```python
from build123d import *

# Parameters (mm, degrees)
SKETCH1_R                = 15
SKETCH1_R_2              = 7.5
BOSS_EXTRUDE1_DEPTH      = 160
BOSS_EXTRUDE1_DEPTH_BACK = 160
SKETCH2_R                = 3.1
CUT_EXTRUDE1_DEPTH       = 16


with BuildPart() as part:
    # Sketch1 → Boss-Extrude1 (new body, two sides)
    with BuildSketch(Plane.XY) as boss_extrude1_sk:
        Circle(SKETCH1_R)
        Circle(SKETCH1_R_2, mode=Mode.SUBTRACT)
    extrude(amount=BOSS_EXTRUDE1_DEPTH)
    extrude(boss_extrude1_sk.sketch, amount=-BOSS_EXTRUDE1_DEPTH_BACK)

    # Sketch2 → Cut-Extrude1 (cut, through all)
    with BuildSketch(Plane(origin=(0, 0, 0), x_dir=(1, 0, 0), z_dir=(0, 1, 0))):
        with Locations((0, -145)):
            Circle(SKETCH2_R)
    cut_extrude1 = extrude(amount=CUT_EXTRUDE1_DEPTH, mode=Mode.SUBTRACT)

    # Mirror1: Cut-Extrude1 across plane
    add(cut_extrude1.mirror(Plane.XY), mode=Mode.SUBTRACT)


solid = part.part
```
The model under review builds one solid part; all positions refer to its coordinate system, in mm. Round coordinates to 2 decimals unless told otherwise and drop trailing zeros. Loops run counter-clockwise (first coordinate to the right, second up) from the corner with the lowest first, then second, coordinate; pieces in that order, holes last. Notation, with made-up numbers: (75, -24.5) -> (123, -24.5) arc R12 ccw to (123, -13.5) -> close; hole circle Ø7 at (48.5, -0.5). An arc over 180 degrees is marked (long way). Answer as a JSON object with one key per item and string values. Group by question number.
1) We need section D-D on z = 145. Write out the cut boundary in (x, y).
2) Mouldability with a two-part tool opening along Z and no side actions: class faces 1 (the face through (-3.1, 10.9, 144.9)), 2 (the face through (-4, 7, 160)), 3 (the face through (-3.1, 10.9, -144.9)), 4 (the face through (-4, 7, -160)) as released by +Z, released by -Z, zero draft, split by the parting line, or undercut.
3) For line 1 (Z direction, x = 0, y = 11); line 2 (Y direction, x = 0, z = 77); line 3 (X direction, y = 8.5, z = -145), list the stretches that pass through material, from the lowest coordinate up. Write a range as [from, to].
4) For pin 1 Ø2 at (x, z) = (2.5, 7.5) entering from -Y; pin 2 Ø3 at (y, z) = (-6.5, -45.5) entering from -X; pin 3 Ø10 at (y, z) = (6.5, -57.5) entering from +X; pin 4 Ø9 at (x, y) = (0, 0) entering from +Z, all flat-tipped, find the tip position at first contact; note any pin that passes through.
5) We need section C-C on z = -126.5. Write out the cut boundary in (x, y).
6) We need section B-B on x = 0. Write out the cut boundary in (y, z).
7) We need section A-A on y = 0. Write out the cut boundary in (x, z), then the cut area to 3 significant figures.
Result set:
{
 "1": {"outline": "(-3.1, 6.83) -> (-3.1, 14.68) arc R15 ccw (long way) to (3.1, 14.68) -> (3.1, 6.83) arc R7.5 cw (long way) to start"},
 "2": {"face 1": "undercut", "face 2": "released by +Z", "face 3": "undercut", "face 4": "released by -Z"},
 "3": {"line 1": "[-160, -148.1], [-141.9, 141.9], [148.1, 160]", "line 2": "[-15, -7.5], [7.5, 15]", "line 3": "[-12.36, -3.1], [3.1, 12.36]"},
 "4": {"pin 1": "y = -14.92", "pin 2": "x = -14.14", "pin 3": "x = 14.92", "pin 4": "through"},
 "5": {"outline": "circle Ø30 at (0, 0); hole circle Ø15 at (0, 0)"},
 "6": {"outline": "(-15, -160) -> (-7.5, -160) -> (-7.5, 160) -> (-15, 160) -> close; (7.5, -160) -> (15, -160) -> (15, -148.1) -> (7.5, -148.1) -> close; (7.5, -141.9) -> (15, -141.9) -> (15, 141.9) -> (7.5, 141.9) -> close; (7.5, 148.1) -> (15, 148.1) -> (15, 160) -> (7.5, 160) -> close"},
 "7": {"outline": "(-15, -160) -> (-7.5, -160) -> (-7.5, 160) -> (-15, 160) -> close; (7.5, -160) -> (15, -160) -> (15, 160) -> (7.5, 160) -> close", "area": "4,800 mm²"}
}
